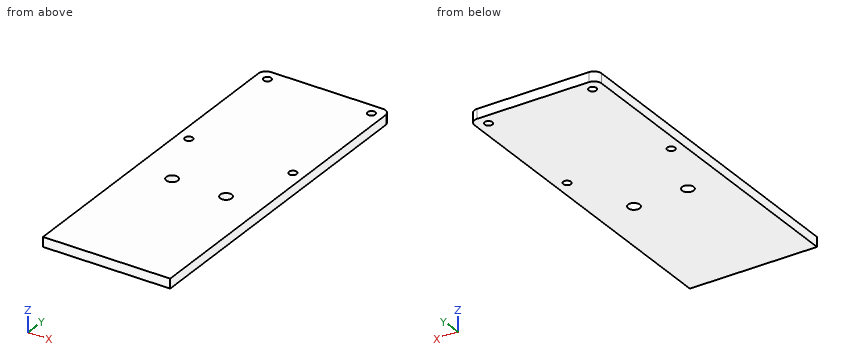
from build123d import *

# Parameters (mm, degrees)
SKETCH1_R           = 1
SKETCH1_R_2         = 1.5
BOSS_EXTRUDE1_DEPTH = 2.5


with BuildPart() as part:
    # Sketch1 → Boss-Extrude1 (new body)
    with BuildSketch(Plane.XY):
        with BuildLine():
            Line((0, 0), (33, 0))
            Line((33, 0), (33, 85))
            ThreePointArc((33, 85), (32.414213562, 86.414213562), (31, 87))
            Line((31, 87), (2, 87))
            ThreePointArc((2, 87), (0.585786438, 86.414213562), (0, 85))
            Line((0, 85), (0, 0))
        make_face()
        with Locations((3, 84)):
            Circle(SKETCH1_R, mode=Mode.SUBTRACT)
        with Locations(Location((3, 53, 0), (0, 0, 180))):
            Circle(SKETCH1_R, mode=Mode.SUBTRACT)
        with Locations((9.5, 36.5)):
            Circle(SKETCH1_R_2, mode=Mode.SUBTRACT)
        with Locations(Location((23.5, 36.5, 0), (0, 0, 180))):
            Circle(SKETCH1_R_2, mode=Mode.SUBTRACT)
        with Locations((30, 53)):
            Circle(SKETCH1_R, mode=Mode.SUBTRACT)
        with Locations(Location((30, 84, 0), (0, 0, 180))):
            Circle(SKETCH1_R, mode=Mode.SUBTRACT)
    extrude(amount=BOSS_EXTRUDE1_DEPTH)


solid = part.part
Geometry check sheet. Reference: the model listing, model coordinates, mm. Give positions to 0.01 mm unless a question says otherwise; leave off trailing zeros. Loops run counter-clockwise (first coordinate to the right, second up) from the corner with the lowest first, then second, coordinate; pieces in that order, holes last. Notation, with made-up numbers: M 59.5,63.5 L 96.5,63.5 A29 ccw 96.5,97.5 Z; hole C 30.25,36.5 d4. An arc over 180 degrees is marked long. Answer as a JSON object with one key per item and string values. Group by question number.
Item 1: Sectioned sample at A-A on y = 36.5. Record the boundary of the cut face in (x, z).
Item 2: Material ranges on L1, parallel to Y at x = 3, z = 1.75; L2, parallel to Y at x = 29.5, z = 1.2; L3, parallel to Y at x = 9.5, z = 1.05, recorded low to high.
Item 3: Sectioned sample at C-C on x = 9.5. Record the boundary of the cut face in (y, z).
Item 4: Sectioned sample at B-B on x = 30. Record the boundary of the cut face in (y, z).
Findings below:
{
 "1": {"outline": "M 0,0 L 8,0 L 8,2.5 L 0,2.5 Z; M 11,0 L 22,0 L 22,2.5 L 11,2.5 Z; M 25,0 L 33,0 L 33,2.5 L 25,2.5 Z"},
 "2": {"L1": "0 to 52, 54 to 83, 85 to 87", "L2": "0 to 52.13, 53.87 to 83.13, 84.87 to 87", "L3": "0 to 35, 38 to 87"},
 "3": {"outline": "M 0,0 L 35,0 L 35,2.5 L 0,2.5 Z; M 38,0 L 87,0 L 87,2.5 L 38,2.5 Z"},
 "4": {"outline": "M 0,0 L 52,0 L 52,2.5 L 0,2.5 Z; M 54,0 L 83,0 L 83,2.5 L 54,2.5 Z; M 85,0 L 87,0 L 87,2.5 L 85,2.5 Z"}
}
